Can you work these out from the model? Positions are in its coordinate system, mm. Give positions to 0.01 mm unless a question says otherwise; leave off trailing zeros. Loops run counter-clockwise (first coordinate to the right, second up) from the corner with the lowest first, then second, coordinate; pieces in that order, holes last. Notation, with made-up numbers: (42.5, -23.5) - (71.5, -23.5) arc R15 ccw to (71.5, 5.5) - close; hole circle Ø1 at (-23.5, 89). An arc over 180 degrees is marked (long way). Use a Markdown table: item, result. Add a question column.
```python
from build123d import *

# Parameters (mm, degrees)
SKETCH1_R          = 6
BASE_FLANGE1_DEPTH = 3


# Sheet-metal steps are written as plain solids
with BuildPart() as part:
    # Sketch1 → Base-Flange1 (new body)
    with BuildSketch(Plane.XY):
        with BuildLine():
            Line((-12.5, 22.5), (-12.5, -22.5))
            ThreePointArc((-12.5, -22.5), (0, -12.044994432), (12.5, -22.5))
            Line((12.5, -22.5), (12.5, 22.5))
            ThreePointArc((12.5, 22.5), (0, 27.67766953), (-12.5, 22.5))
        make_face()
        with Locations((0, 10)):
            Circle(SKETCH1_R, mode=Mode.SUBTRACT)
    extrude(amount=-BASE_FLANGE1_DEPTH)


solid = part.part
```
1. Suppose I cut it at B-B (z = -0.75). List the corners of the cut face in (x, y) for me (3 decimals).
2. Will these pins go through, and if not, where does the flat tip stop? P1, Ø1, axis at x = -7.5, z = -1, coming from the +Y side; P2, Ø9.5, axis at x = 0, y = 10, coming from the -Z side.
3. Please list where these lines run through material, in increasing order: line 1 along Y through (x, z) = (0, -2.2) (3 decimals); line 2 along X through (y, z) = (8.5, -2.25); line 3 along X through (y, z) = (-18.5, -2.7). Write a range as [from, to].
4. Suppose I cut it at A-A (x = 0). List the corners of the cut face in (y, z) for me (3 decimals).
5. Suppose I cut it at C-C (y = -14). List the corners of the cut face in (x, z) for me, and give its area (3 significant figures).
6. Suppose I cut it at D-D (x = 10.5). List the corners of the cut face in (y, z) for me, and give its area (3 significant figures).
7. If we mould it in two halves opening along Y, with no side actions, what happens to faces 1 (the face through (12.5, 0, -1)), 2 (the face through (-1.301, 4.143, -1.479)), 3 (the face through (0.194, 27.677, -1.479))? For each: released by +Y, released by -Y, zero draft, split by the parting line, or undercut.
Results below:
| question | item | result |
|---|---|---|
| 1 | outline | (-12.5, -22.5) arc R12.7 cw to (12.5, -22.5) - (12.5, 22.5) arc R17.678 ccw to (-12.5, 22.5) - close; hole circle Ø12 at (0, 10) |
| 2 | P1 | y = 26.23 |
| 2 | P2 | through |
| 3 | line 1 | [-12.045, 4], [16, 27.678] |
| 3 | line 2 | [-12.5, -5.81], [5.81, 12.5] |
| 3 | line 3 | [-12.5, -11.06], [11.06, 12.5] |
| 4 | outline | (-12.045, -3) - (4, -3) - (4, 0) - (-12.045, 0) - close; (16, -3) - (27.678, -3) - (27.678, 0) - (16, 0) - close |
| 5 | outline | (-12.5, -3) - (-6.77, -3) - (-6.77, 0) - (-12.5, 0) - close; (6.77, -3) - (12.5, -3) - (12.5, 0) - (6.77, 0) - close |
| 5 | area | 34.4 mm² |
| 6 | outline | (-17.6, -3) - (24.22, -3) - (24.22, 0) - (-17.6, 0) - close |
| 6 | area | 125 mm² |
| 7 | face 1 | zero draft |
| 7 | face 2 | undercut |
| 7 | face 3 | released by +Y |
